Geometry check sheet. Reference: the model listing, model coordinates, mm. A direction names the side the tool comes from. Give positions to 0.01 mm unless a question says otherwise; leave off trailing zeros. Loops run counter-clockwise (first coordinate to the right, second up) from the corner with the lowest first, then second, coordinate; pieces in that order, holes last. Notation, with made-up numbers: (-2, 20.5) - (18, 20.5) arc R23 cw to (18, 31.5) - close; hole circle Ø11 at (-17.75, 68.25). An arc over 180 degrees is marked (long way). One line per question, with ' | ' between items. Start each with the question number.
Autodesk Inventor part; units mm, degrees
ref_plane "YZ Plane" through (0, 0, 0) normal (1, 0, 0) x (0, 1, 0)
ref_plane "XZ Plane" through (0, 0, 0) normal (0, 1, 0) x (-1, 0, 0)
ref_plane "XY Plane" through (0, 0, 0) normal (0, 0, 1) x (1, 0, 0)
sketch "Sketch1" plane through (0, 0, 0) normal (0, 1, 0) x (-1, 0, 0)
  line L0 (25, 0) -> (25, 45)
  line L1 (25, 45) -> (-25, 45)
  line L2 (-25, 45) -> (-25, 0)
  line L3 (25, 0) -> (-25, 0)
  line L4 (20, 5) -> (-20, 5)
  line L5 (-20, 5) -> (-20, 40)
  line L6 (-20, 40) -> (20, 40)
  line L7 (20, 40) -> (20, 5)
  point P0 (0, 0)
  dimension "d2" = 45
  dimension "d3" = 50
  dimension "d4" = 45
  dimension "d5" = 50
  dimension "d9" = 35
  dimension "d10" = 40
  dimension "d11" = 35
extrude "Extrusion1" add sketch "Sketch1" along normal blind 6
sketch "Sketch2" plane through (0, 0, 0) normal (0, -1, 0) x (1, 0, 0)
  line L0 (25, 45) -> (25, 0)
  line L1 (-25, 45) -> (25, 45)
  circle A0 centre (22.5, 33.5) radius 2.5
  line L2 (-25, 0) -> (-25, 45)
  line L3 (25, 0) -> (-25, 0)
  circle A1 centre (-22.5, 11.5) radius 2.5
  point P0 (0, 0)
  dimension "d16" = 5
  dimension "d19" = 5
extrude "Extrusion2" add sketch "Sketch2" along normal blind 7.5 contours A1 | A0
sketch "Sketch3" plane through (22.5, -7.5, 33.5) normal (0, -1, 0) x (1, 0, 0)
  circle A0 centre (0, 0) radius 3.5
  point P0 (-22.5, -33.5)
  dimension "d22" = 7
sketch "Sketch4" plane through (-22.5, -7.5, 11.5) normal (0, -1, 0) x (1, 0, 0)
  circle A0 centre (0, 0) radius 3.5
  point P0 (22.5, -11.5)
  dimension "d23" = 7
extrude "Extrusion3" add sketch "Sketch4" along normal blind 2
extrude "Extrusion4" add sketch "Sketch3" along normal blind 2
sketch "Sketch6" plane through (25, 0, 0) normal (1, 0, 0) x (0, 0, -1)
  line L0 (0, 0) -> (0, 6)
  line L1 (0, 0) -> (0, 6)
  line L2 (-45, 0) -> (-45, 6)
  circle A0 centre (-42, 3) radius 2
  circle A1 centre (-3, 3) radius 2
  dimension "d41" = 6
  dimension "d44" = 4
  dimension "d45" = 4
hole "Hole2" at (25, 3, 42) at (25, 3, 3) direction (-1, 0, 0) diameter 4 end through all both
(1) Mould release check, pull along Z, two halves, no side actions. Record for faces 1 (the face through (8, 0, 3)), 2 (the face through (0, 2, 5)), 3 (the face through (0, 5, 3)), 4 (the face through (-20.885, -8.486, 14.605)): pulls with the +Z half, pulls with the -Z half, needs draft (parallel to the pull), parting line crosses it, or undercut.
(2) Material ranges on line 1 (Y direction, x = 0, z = 3); line 2 (X direction, y = 5, z = 7); line 3 (Z direction, x = 23, y = 2.5), recorded low to high.
(3) Section check B-B, the plane z = 3. Record the boundary of the cut face in (x, y), and give its area (3 significant figures).
(4) Section check D-D, the plane z = 18.5. Record the boundary of the cut face in (x, y), and give its area (3 significant figures).
(5) Depth check by flat-ended pin: pin 1 Ø6.5 at (y, z) = (4.5, 18.5) entering from -X; pin 2 Ø10 at (x, z) = (7, 8.5) entering from -Y; pin 3 Ø6.5 at (y, z) = (3, 3) entering from +X; pin 4 Ø3 at (y, z) = (-6.5, 6.5) entering from +X. Enter the tip coordinate at first touch or a pass-through.
(6) Section check C-C, the plane x = 22.5. Record the boundary of the cut face in (y, z).
(7) Tool access check on faces 5 (the face through (-21, -7.5, 9)), 6 (the face through (0, 1, 40)), 7 (the face through (0, 3, 0)), 8 (the face through (25, 3, 23)), 9 (the face through (-25, 3, 22)). Record the directions out of +Z, -Z, +X, -X, +Y, -Y that give a thin tool (end or side, any length) a straight path to the whole face; none if there is none.
Numbers:
1) face 1: needs draft | face 2: undercut | face 3: undercut | face 4: parting line crosses it
2) line 1: 0 to 1, 5 to 6 | line 2: -25 to -20, 20 to 25 | line 3: 0 to 1.06, 4.94 to 40.06, 43.94 to 45
3) outline: (-25, 0) - (25, 0) - (25, 1) - (-25, 1) - close; (-25, 5) - (25, 5) - (25, 6) - (-25, 6) - close | area: 100 mm^2
4) outline: (-25, 0) - (-20, 0) - (-20, 6) - (-25, 6) - close; (20, 0) - (25, 0) - (25, 6) - (20, 6) - close | area: 60.0 mm^2
5) pin 1: x = -25 | pin 2: y = 0 | pin 3: x = 25 | pin 4: through
6) outline: (-9.5, 30) - (-7.5, 30) - (-7.5, 31) - (0, 31) - (0, 0) - (6, 0) - (6, 45) - (0, 45) - (0, 36) - (-7.5, 36) - (-7.5, 37) - (-9.5, 37) - close; hole circle Ø4 at (3, 3); hole circle Ø4 at (3, 42)
7) face 5: none | face 6: +Y, -Y | face 7: -Z, +X, -X, +Y, -Y | face 8: +Z, -Z, +X, +Y | face 9: +Z, -Z, -X, +Y
